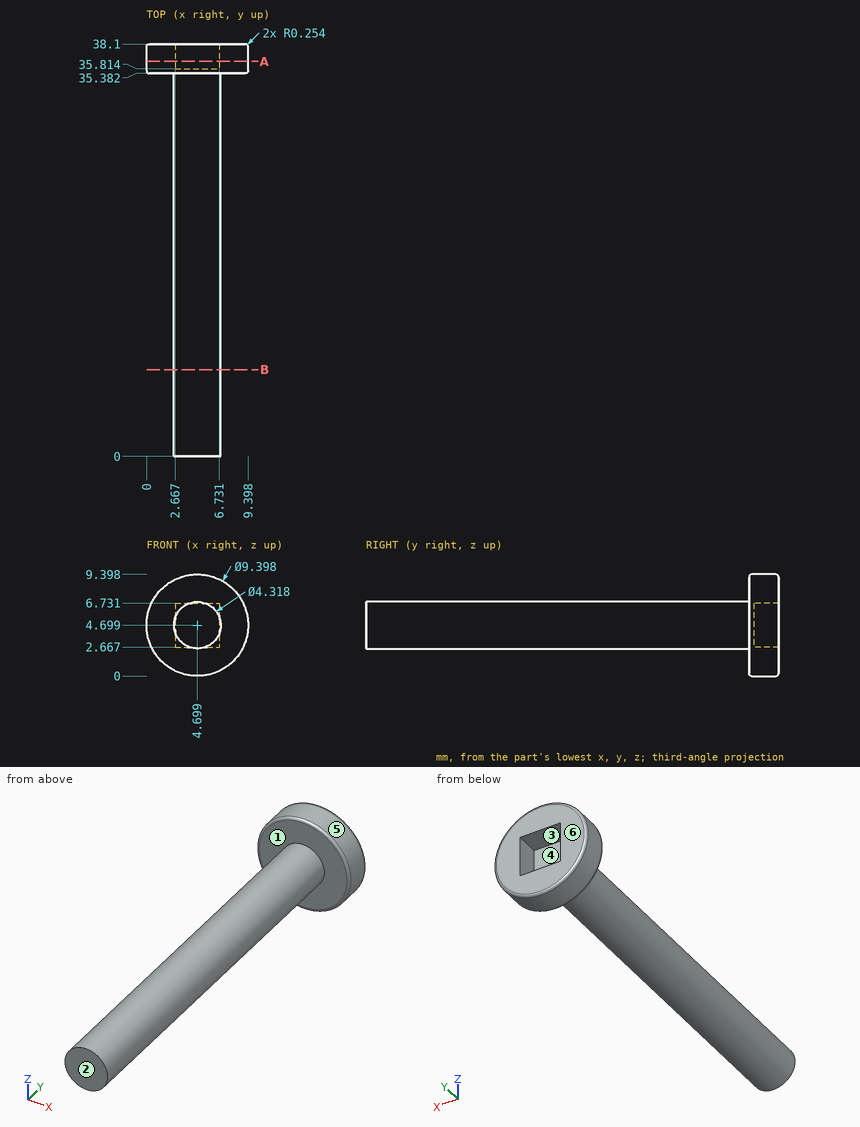
Answer from the drawing. Dimensions are ordinates in mm from the lowest x, y and z of the part. A direction names the side the tool comes from. Give positions to 0.01 mm unless a question says otherwise; leave off trailing zeros. Loops run counter-clockwise (first coordinate to the right, second up) from the corner with the lowest first, then second, coordinate; pieces in that order, holes last.
Item 1: A tool of negligible diameter and unlimited length cuts with its end or side. For the marked faces 1 and 2, from which of +Z, -Z, +X, -X, +Y, -Y can it reach the whole face along a straight path? Write none if from no direction.
Derived:
face 1: -Y
face 2: +Z, -Z, +X, -X, -Y
Item 2: Each of these flat-tipped pins is pushed along its axis until it touches: pin 1 Ø1 at (x, z) = (3.5, 2) entering from -Y; pin 2 Ø1.1 at (x, y) = (5.5, 37.5) entering from +Z; pin 3 Ø4 at (x, y) = (5.5, 31) entering from -Z. Where does it stop, or does it pass through?
Derived:
pin 1: stops at y = 35.38
pin 2: stops at z = 9.39
pin 3: stops at z = 2.54
Item 3: A cutting plane is placed at B-B (y = 8). Give the vertices of the cut face in (x, z).
Derived:
outline: circle Ø4.32 at (4.7, 4.7)
Item 4: Determine the mould class of the marked faces 3, 4, 5 and 6 for opening direction X: +X half, -X half, draft (parallel to the pull), parting line (faces both ways), or undercut.
Derived:
face 3: undercut
face 4: undercut
face 5: parting line
face 6: draft
Item 5: A cutting plane is placed at A-A (y = 36.5). Give the vertices of the cut face in (x, z).
Derived:
outline: circle Ø9.4 at (4.7, 4.7); hole (2.67, 2.67) - (6.73, 2.67) - (6.73, 6.73) - (2.67, 6.73) - close
Item 6: Find the intervals of material crossed by line 1 along Z through (x, y) = (4.5, 36.5); line 2 along Y through (x, z) = (3.25, 3); line 3 along Y through (x, z) = (5, 4), in increasing order.
Derived:
line 1: z = 0 to 2.67, 6.73 to 9.39
line 2: y = 35.38 to 35.81
line 3: y = 0 to 35.81
